```python
from build123d import *

# Parameters (mm, degrees)
SKETCH_R      = 1.5
SKETCH_R_2    = 1
PAD_DEPTH     = 5
SKETCH001_R   = 6
SKETCH001_R_2 = 1.5
PAD001_DEPTH  = 3


with BuildPart() as part:
    # Sketch → Pad (new body)
    with BuildSketch(Plane.XY):
        with BuildLine():
            ThreePointArc((-45, 6), (-51, 0), (-45, -6))
            Line((-45, -6), (0, -6))
            Line((0, -6), (0, 6))
            Line((-45, 6), (0, 6))
        make_face()
        with Locations((-45, 0)):
            Circle(SKETCH_R, mode=Mode.SUBTRACT)
        with Locations((-15.5, 0)):
            Circle(SKETCH_R_2, mode=Mode.SUBTRACT)
    extrude(amount=PAD_DEPTH)

    # Sketch001 (on Face8 of Pad) → Pad001 (join)
    with BuildSketch(Plane.XY.offset(5)):
        with Locations((-45, 0)):
            Circle(SKETCH001_R)
        with Locations((-45, 0)):
            Circle(SKETCH001_R_2, mode=Mode.SUBTRACT)
    extrude(amount=PAD001_DEPTH)

    # Mirrored: part across Sketch001 V_Axis


with BuildPart() as part_1:
    add(part.part)
    add(part.part.mirror(Plane(origin=(0, 0, 5), x_dir=(0, 0, 1), z_dir=(1, 0, 0))))


solid = part_1.part
```
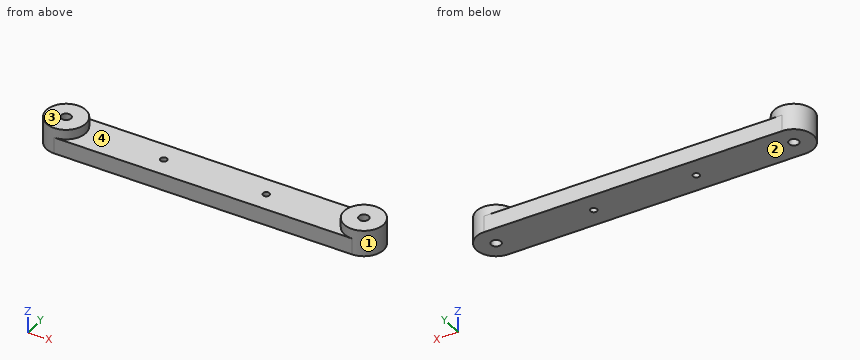
CAD build for the part. Positions are in the model's coordinates, mm. Face numbers are marked on the shaded views. A direction names the side the tool comes from. Coordinates: 2 decimals unless noted, no trailing zeros. Order: outer loops, then holes, each group sorted by start corner. A loop starts at its lowest first (then second) coordinate and runs counter-clockwise, first axis right, second up. Notation, with made-up numbers: (45.25, 17) - (68.25, 17) arc R35 ccw to (68.25, 49) - close; hole circle Ø2 at (18, -9). An arc over 180 degrees is marked (long way). Use a Markdown table: item, result. Add a question column.
(1) Saw through at B-B (x = -15.5). Give the cut face in (y, z), then the cut area to 3 significant figures.
(2) Saw through at C-C (z = 3). Give the cut face in (x, y), then the cut area to 3 significant figures.
(3) Drill centre lines: line 1 along Y through (x, z) = (-15.5, 2.7); line 2 along Y through (x, z) = (45, 3.5); line 3 along X through (y, z) = (-0.25, 4). Where is each one in solid material? Low to high. Write a range as [from, to].
(4) Saw through at D-D (y = 4.75). Give the cut face in (x, z).
(5) Pull direction X, two halves, no side cores. Call the marked faces 3 and 4: +X half, -X half, draft (parallel to the pull), parting line (faces both ways), or undercut.
(6) Which spindle directions (+Z, -Z, +X, -X, +Y, -Y) get a long thin tool onto all of the face, cutting with end or side? Do the marked faces 1 and 2. Say none if no direction does.
(7) Saw through at A-A (y = 0). Give the cut face in (x, z).
(8) Flat gauge pins, fed straight in: pin 1 (1.8 mm diameter, centred on x = -45, y = 0, fed in from +Z); pin 2 (1 mm diameter, centred on y = -4.5, z = 4.5, fed in from -X); pin 3 (4 mm diameter, centred on y = 2.5, z = 4, fed in from +X); pin 4 (2.5 mm diameter, centred on x = -15.5, y = 0, fed in from +Z). Where does each tip first touch, or does it go through?
Solved:
| question | item | result |
|---|---|---|
| 1 | outline | (-6, 0) - (-1, 0) - (-1, 5) - (-6, 5) - close; (1, 0) - (6, 0) - (6, 5) - (1, 5) - close |
| 1 | area | 50.0 mm² |
| 2 | outline | (-45, -6) - (45, -6) arc R6 ccw to (45, 6) - (-45, 6) arc R6 ccw to start; hole circle Ø3 at (-45, 0); hole circle Ø2 at (-15.5, 0); hole circle Ø2 at (15.5, 0); hole circle Ø3 at (45, 0) |
| 2 | area | 1,170 mm² |
| 3 | line 1 | y = [-6, -1], [1, 6] |
| 3 | line 2 | y = [-6, -1.5], [1.5, 6] |
| 3 | line 3 | x = [-50.99, -46.48], [-43.52, -16.47], [-14.53, 14.53], [16.47, 43.52], [46.48, 50.99] |
| 4 | outline | (-48.67, 0) - (48.67, 0) - (48.67, 8) - (41.33, 8) - (41.33, 5) - (-41.33, 5) - (-41.33, 8) - (-48.67, 8) - close |
| 5 | face 3 | draft |
| 5 | face 4 | undercut |
| 6 | face 1 | +Z |
| 6 | face 2 | -Z, +X, -X, +Y, -Y |
| 7 | outline | (-51, 0) - (-46.5, 0) - (-46.5, 8) - (-51, 8) - close; (-43.5, 0) - (-16.5, 0) - (-16.5, 5) - (-39, 5) - (-39, 8) - (-43.5, 8) - close; (-14.5, 0) - (14.5, 0) - (14.5, 5) - (-14.5, 5) - close; (16.5, 0) - (43.5, 0) - (43.5, 8) - (39, 8) - (39, 5) - (16.5, 5) - close; (46.5, 0) - (51, 0) - (51, 8) - (46.5, 8) - close |
| 8 | pin 1 | passes through |
| 8 | pin 2 | stops at x = -49.47 |
| 8 | pin 3 | stops at x = 50.98 |
| 8 | pin 4 | stops at z = 5 |
